Verification items for this drawing (mm, ordinates from the low corner). Coordinates: 2 decimals unless noted, no trailing zeros. Order: outer loops, then holes, each group sorted by start corner. A loop starts at its lowest first (then second) coordinate and runs counter-clockwise, first axis right, second up. Notation, with made-up numbers: (15, 22.5) -> (52, 22.5) arc R31 ccw to (52, 48.5) -> close; hole circle Ø10 at (2, -23.75). An arc over 180 degrees is marked (long way). Answer in a Markdown table with one row per item. Add a question column.
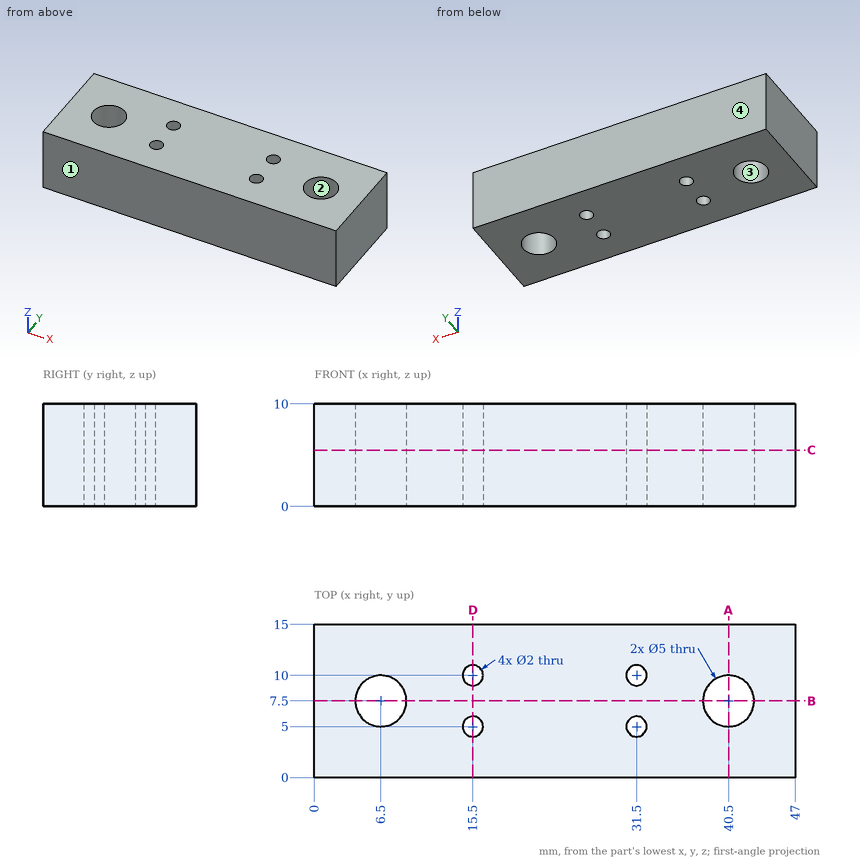
(1) Cross-section at C-C (z = 5.5). Enter the section's corners in (x, y), plus the area to 3 significant figures.
(2) Mould release check, pull along Y, two halves, no side actions. Record for the marked faces 1, 2, 3 and 4: +Y half, -Y half, draft (parallel to the pull), parting line (faces both ways), or undercut.
(3) Go/stop test with a flat-tipped pin: P1, Ø1.2, axis at x = 15.5, y = 10, coming from the +Z side. Record where the tip stops, or that it passes through.
(4) Cross-section at B-B (y = 7.5). Enter the section's corners in (x, z).
(5) Scan lines: line 1 along Y through (x, z) = (15.5, 3); line 2 along Y through (x, z) = (6.5, 6); line 3 along Y through (x, z) = (4.5, 3). Record each from-to range of solid material in increasing order.
(6) Cross-section at A-A (x = 40.5). Enter the section's corners in (y, z).
(7) Cross-section at D-D (x = 15.5). Enter the section's corners in (y, z), plus the area to 3 significant figures.
Checks:
| question | item | result |
|---|---|---|
| 1 | outline | (0, 0) -> (47, 0) -> (47, 15) -> (0, 15) -> close; hole circle Ø5 at (6.5, 7.5); hole circle Ø2 at (15.5, 5); hole circle Ø2 at (15.5, 10); hole circle Ø2 at (31.5, 5); hole circle Ø2 at (31.5, 10); hole circle Ø5 at (40.5, 7.5) |
| 1 | area | 653 mm² |
| 2 | face 1 | -Y half |
| 2 | face 2 | undercut |
| 2 | face 3 | undercut |
| 2 | face 4 | +Y half |
| 3 | P1 | through |
| 4 | outline | (0, 0) -> (4, 0) -> (4, 10) -> (0, 10) -> close; (9, 0) -> (38, 0) -> (38, 10) -> (9, 10) -> close; (43, 0) -> (47, 0) -> (47, 10) -> (43, 10) -> close |
| 5 | line 1 | 0 to 4, 6 to 9, 11 to 15 |
| 5 | line 2 | 0 to 5, 10 to 15 |
| 5 | line 3 | 0 to 6, 9 to 15 |
| 6 | outline | (0, 0) -> (5, 0) -> (5, 10) -> (0, 10) -> close; (10, 0) -> (15, 0) -> (15, 10) -> (10, 10) -> close |
| 7 | outline | (0, 0) -> (4, 0) -> (4, 10) -> (0, 10) -> close; (6, 0) -> (9, 0) -> (9, 10) -> (6, 10) -> close; (11, 0) -> (15, 0) -> (15, 10) -> (11, 10) -> close |
| 7 | area | 110 mm² |
